For this review, take the finished solid that the model builds, in its own axes (mm). A direction names the side the tool comes from. Coordinates: 2 decimals unless noted, no trailing zeros. Order: outer loops, then holes, each group sorted by start corner. A loop starts at its lowest first (then second) coordinate and runs counter-clockwise, first axis right, second up.
from build123d import *

# Parameters (mm, degrees)
CYLINDER112024025003003006010004028_R     = 1.7
CYLINDER112024025003003006010004028_DEPTH = 14
CYLINDER112024025003003006010004021_R     = 1.15
CYLINDER112024025003003006010004021_DEPTH = 14
CYLINDER112024025003003006010004027_R     = 4.3
CYLINDER112024025003003006010004027_DEPTH = 14
CYLINDER112024025003003006010004043_R     = 1
CYLINDER112024025003003006010004043_DEPTH = 14
BOX021079_W                               = 8
BOX021079_H                               = 8.6
BOX021079_DEPTH                           = 14
CHAMFER008_SIZE                           = 0.3


with BuildPart() as obj1:
    # Cylinder112024025003003006010004028 → Cylinder112024025003003006010004028 (new body)
    with BuildSketch(Plane(origin=(17.5, -24, 11), x_dir=(0, 0, -1), z_dir=(1, 0, 0))):
        Circle(CYLINDER112024025003003006010004028_R)
    extrude(amount=CYLINDER112024025003003006010004028_DEPTH)


with BuildPart() as fusion005043005007002015:
    # Cylinder112024025003003006010004021 → Cylinder112024025003003006010004021 (new body)
    with BuildSketch(Plane(origin=(14, -24, 6), x_dir=(1, 0, 0), z_dir=(0, 0, 1))):
        Circle(CYLINDER112024025003003006010004021_R)
    extrude(amount=CYLINDER112024025003003006010004021_DEPTH)

    # Fusion005043005007002015: union obj1
    add(obj1.part)


with BuildPart() as obj2:
    # Cylinder112024025003003006010004027 → Cylinder112024025003003006010004027 (new body)
    with BuildSketch(Plane(origin=(10, -24, 6), x_dir=(1, 0, 0), z_dir=(0, 0, 1))):
        Circle(CYLINDER112024025003003006010004027_R)
    extrude(amount=CYLINDER112024025003003006010004027_DEPTH)


with BuildPart() as obj3:
    # Cylinder112024025003003006010004043 → Cylinder112024025003003006010004043 (new body)
    with BuildSketch(Plane(origin=(11, -24, 4), x_dir=(1, 0, 0), z_dir=(0, 0, 1))):
        Circle(CYLINDER112024025003003006010004043_R)
    extrude(amount=CYLINDER112024025003003006010004043_DEPTH)


with BuildPart() as tensioner:
    # Box021079 → Box021079 (new body)
    with BuildSketch(Plane(origin=(10, -28.3, 6), x_dir=(1, 0, 0), z_dir=(0, 0, 1))):
        with Locations((4, 4.3)):
            Rectangle(BOX021079_W, BOX021079_H)
    extrude(amount=BOX021079_DEPTH)

    # Fusion005043005007002014: union obj2, obj3
    add(obj2.part)
    add(obj3.part)

    # Cut018020020009027020002003004004013: cut Fusion005043005007002015
    add(fusion005043005007002015.part, mode=Mode.SUBTRACT)

    # Chamfer008
    chamfer008_edges = [tensioner.edges().sort_by_distance(p)[0] for p in [
        (18, -28.3, 13),
        (18, -19.7, 13),
    ]]
    chamfer(chamfer008_edges, length=CHAMFER008_SIZE)


solid = tensioner.part
1. Clearance check with flat-ended pins moving along their axes: pin 1 Ø3 at (x, z) = (7.5, 11) entering from +Y; pin 2 Ø3 at (y, z) = (-22, 13.5) entering from -X; pin 3 Ø2.5 at (x, y) = (14, -24) entering from -Z. State where each tip first meets the part, or that it passes through.
Answer below:
pin 1: stops at y = -19.82
pin 2: stops at x = 5.73
pin 3: stops at z = 6
2. Machinability: for faces 4 (the face through (11, -25, 5)), 5 (the face through (14, -28.3, 13)), 6 (the face through (17.5, -24, 11)), which of the approach directions +Z, -Z, +X, -X, +Y, -Y give a long, thin tool a straight path to every point of the face, cutting with its end or side? Answer none if there is none.
Answer below:
face 4: -Z
face 5: +Z, -Z, +X, -X, -Y
face 6: +X
3. Take a section at A-A, the plane z = 16.25. Give the boundary of the cut face in (x, y), plus the area to 3 significant figures.
Answer below:
outline: (10, -28.3) - (17.7, -28.3) - (18, -28) - (18, -20) - (17.7, -19.7) - (10, -19.7) arc R4.3 ccw to start; hole circle Ø2.3 at (14, -24)
area: 93.6 mm2
4. The part is to be moulded in two halves that separate along X. For faces 1 (the face through (5.7, -23.9, 12.9)), 2 (the face through (13.751, -25.123, 12.902)), 3 (the face through (12, -24, 20)), say which applies: +X half, -X half, draft (parallel to the pull), parting line (faces both ways), or undercut.
Answer below:
face 1: -X half
face 2: undercut
face 3: draft
5. Take a section at C-C, the plane x = 14. Give the boundary of the cut face in (y, z), plus the area to 3 significant figures.
Answer below:
outline: (-28.3, 6) - (-25.15, 6) - (-25.15, 20) - (-28.3, 20) - close; (-22.85, 6) - (-19.7, 6) - (-19.7, 20) - (-22.85, 20) - close
area: 88.2 mm2
6. Take a section at B-B, the plane y = -24. Give the boundary of the cut face in (x, z).
Answer below:
outline: (5.7, 6) - (10, 6) - (10, 4) - (12, 4) - (12, 6) - (12.85, 6) - (12.85, 20) - (5.7, 20) - close; (15.15, 6) - (18, 6) - (18, 9.3) - (17.5, 9.3) - (17.5, 12.7) - (18, 12.7) - (18, 20) - (15.15, 20) - close
7. Take a section at D-D, the plane x = 11. Give the boundary of the cut face in (y, z), plus the area to 3 significant figures.
Answer below:
outline: (-28.3, 6) - (-25, 6) - (-25, 4) - (-23, 4) - (-23, 6) - (-19.7, 6) - (-19.7, 20) - (-28.3, 20) - close
area: 124 mm2
8. To check wall thickness, follow L1, parallel to Z at x = 17.9, y = -24; L2, parallel to Y at x = 14, z = 10.5; L3, parallel to Z at x = 13, y = -20.75. State the ranges of each line that lie inside material, in increasing order.
Answer below:
L1: z = 6 to 9.3, 12.7 to 20
L2: y = -28.3 to -25.15, -22.85 to -19.7
L3: z = 6 to 20
